Here's how the part is built. I have some questions about the finished solid (model axes, mm). A direction names the side the tool comes from. Give positions to 0.01 mm unless a question says otherwise; leave off trailing zeros. Write each loop counter-clockwise with the first axis right and the second up, starting at its lowest first coordinate (ties: lowest second). Pieces come first, ordered by that corner, then holes. Notation, with made-up numbers: (-28.5, 2.25) -> (-7.5, 2.25) arc R7 cw to (-7.5, 11.25) -> close; hole circle Ø8 at (70.25, 89). An arc over 180 degrees is marked (long way). Use one line per item in the form item = value.
```python
from build123d import *

# Parameters (mm, degrees)
IZIM2_R                     = 6
Y_KSEKLIK_EKSTR_ZYON2_DEPTH = 12
IZIM4_R                     = 25
IZIM4_R_2                   = 13
Y_KSEKLIK_EKSTR_ZYON3_DEPTH = 62
IZIM4_6_R                   = 25
IZIM4_6_R_2                 = 13
Y_KSEKLIK_EKSTR_ZYON4_DEPTH = 19
IZIM5_R                     = 25
IZIM5_R_2                   = 13
Y_KSEKLIK_EKSTR_ZYON5_DEPTH = 19


with BuildPart() as part:
    # Çizim2 → Yükseklik-Ekstrüzyon2 (new body)
    with BuildSketch(Plane.XY):
        with BuildLine():
            Line((17.332096605, 35.875327714), (62.829976007, 130.050393256))
            ThreePointArc((62.829976007, 130.050393256), (89.842699599, 147), (116.85542319, 130.050393256))
            Line((116.85542319, 130.050393256), (162.353302592, 35.875327714))
            ThreePointArc((162.353302592, 35.875327714), (161.019139253, 11.712471879), (139.842699599, 0))
            Line((139.842699599, 0), (39.842699599, 0))
            ThreePointArc((39.842699599, 0), (18.666259945, 11.712471879), (17.332096605, 35.875327714))
        make_face()
        with Locations((89.842699599, 117)):
            Circle(IZIM2_R, mode=Mode.SUBTRACT)
        with Locations((39.842699599, 25)):
            Circle(IZIM2_R, mode=Mode.SUBTRACT)
        with Locations((139.842699599, 25)):
            Circle(IZIM2_R, mode=Mode.SUBTRACT)
    extrude(amount=Y_KSEKLIK_EKSTR_ZYON2_DEPTH)

    # Çizim4 → Yükseklik-Ekstrüzyon3 (add)
    with BuildSketch(Plane(origin=(0, 25, 0), x_dir=(-1, 0, 0), z_dir=(0, -1, 0))):
        with BuildLine():
            ThreePointArc((-107.851357607, -42), (-92.851357607, -37), (-77.851357607, -42))
            Line((-77.851357607, -42), (-77.851357607, -12))
            Line((-77.851357607, -12), (-107.851357607, -12))
            Line((-107.851357607, -12), (-107.851357607, -42))
        make_face()
        with Locations((-92.851357607, -62)):
            Circle(IZIM4_R)
        with Locations(Location((-92.851357607, -62, 0), (0, 0, 90))):
            Circle(IZIM4_R_2, mode=Mode.SUBTRACT)
    extrude(amount=-Y_KSEKLIK_EKSTR_ZYON3_DEPTH)

    # Çizim4<6> → Yükseklik-Ekstrüzyon4 (add)
    with BuildSketch(Plane(origin=(0, 25, 0), x_dir=(-1, 0, 0), z_dir=(0, -1, 0))):
        with Locations(Location((-92.851357607, -62, 0), (0, 0, 90))):
            Circle(IZIM4_6_R)
        with Locations(Location((-92.851357607, -62, 0), (0, 0, 90))):
            Circle(IZIM4_6_R_2, mode=Mode.SUBTRACT)
    extrude(amount=Y_KSEKLIK_EKSTR_ZYON4_DEPTH)

    # Çizim5 → Yükseklik-Ekstrüzyon5 (add)
    with BuildSketch(Plane(origin=(0, 87, 0), x_dir=(1, 0, 0), z_dir=(0, 1, 0))):
        with Locations(Location((92.851357607, -62, 0), (0, 0, 90))):
            Circle(IZIM5_R)
        with Locations(Location((92.851357607, -62, 0), (0, 0, 90))):
            Circle(IZIM5_R_2, mode=Mode.SUBTRACT)
    extrude(amount=Y_KSEKLIK_EKSTR_ZYON5_DEPTH)


solid = part.part
```
Q1. Will these pins go through, and if not, where does the flat tip stop? pin 1 Ø4 at (y, z) = (57, 44.5) entering from +X; pin 2 Ø9 at (y, z) = (47, 32.5) entering from +X; pin 3 Ø24 at (x, z) = (88.5, 32) entering from -Y.
Result set:
pin_1 = 112.47
pin_2 = 107.85
pin_3 = 6
Q2. I want a section at B-B, the plane z = 8. Write out the boundary of the cut face in (x, y), and give its area (3 significant figures).
Result set:
outline = (17.33, 35.88) arc R25 ccw to (39.84, 0) -> (139.84, 0) arc R25 ccw to (162.35, 35.88) -> (116.86, 130.05) arc R30 ccw to (62.83, 130.05) -> close; hole circle Ø12 at (39.84, 25); hole circle Ø12 at (89.84, 117); hole circle Ø12 at (139.84, 25)
area = 14,800 mm2
Q3. If I drill on line 1 along X through (y, z) = (66, 62); line 2 along Z through (x, y) = (88, 99.5); line 3 along Z through (x, y) = (94.5, 15.5), over which ranges is the centre line in solid material (lowest first)? Write a range as from..to.
Result set:
line_1 = 67.85..79.85, 105.85..117.85
line_2 = 0..12, 37.48..49.94, 74.06..86.52
line_3 = 0..12, 37.05..49.1, 74.9..86.95
Q4. I want a section at D-D, the plane x = 91. Write out the boundary of the cut face in (y, z).
Result set:
outline = (0, 0) -> (111.11, 0) -> (111.11, 12) -> (87, 12) -> (87, 37.07) -> (106, 37.07) -> (106, 49.13) -> (6, 49.13) -> (6, 37.07) -> (25, 37.07) -> (25, 12) -> (0, 12) -> close; (6, 74.87) -> (106, 74.87) -> (106, 86.93) -> (6, 86.93) -> close; (122.89, 0) -> (146.98, 0) -> (146.98, 12) -> (122.89, 12) -> close
Q5. I want a section at A-A, the plane z = 62. Write out the boundary of the cut face in (x, y).
Result set:
outline = (67.85, 6) -> (79.85, 6) -> (79.85, 106) -> (67.85, 106) -> close; (105.85, 6) -> (117.85, 6) -> (117.85, 106) -> (105.85, 106) -> close
Q6. I want a section at C-C, the plane y = 117. Write out the boundary of the cut face in (x, z).
Result set:
outline = (56.53, 0) -> (83.84, 0) -> (83.84, 12) -> (56.53, 12) -> close; (95.84, 0) -> (123.16, 0) -> (123.16, 12) -> (95.84, 12) -> close
Q7. If we mould it in two halves opening along X, with no side actions, what happens to faces 1 (the face through (33.85, 25.26, 5.92)), 2 (the face through (161.205, 12.013, 5.916)), 3 (the face through (82, 6, 51))? For each: +X half, -X half, draft (parallel to the pull), parting line (faces both ways), or undercut.
Result set:
face_1 = undercut
face_2 = +X half
face_3 = draft
Q8. Which directions (+Z, -Z, +X, -X, +Y, -Y) give clear straight access to the entire face, cutting with the end or side of a thin tool? Please do faces 4 (the face through (77.851, 56, 27)), 5 (the face through (107.851, 56, 27)), 6 (the face through (89.372, 146.996, 5.916)), 7 (the face through (104, 106, 51)).
Result set:
face_4 = -X, +Y, -Y
face_5 = +X, +Y, -Y
face_6 = +Z, -Z, +Y
face_7 = +Z, +X, -X, +Y
